from build123d import *

# Parameters (mm, degrees)
SKETCH_1_W          = 12
SKETCH_1_H          = 12
EXTRUDE_1_DEPTH     = 12
SKETCH_2_R          = 2
CUT_EXTRUDE_1_DEPTH = 21.784609691
SKETCH_3_R          = 2
CUT_EXTRUDE_2_DEPTH = 21.784609691
SKETCH_4_R          = 2
CUT_EXTRUDE_3_DEPTH = 21.784609691


with BuildPart() as part:
    # 草图1 → 凸台-拉伸1 (new body)
    with BuildSketch(Plane.XY):
        with Locations((6, -6)):
            Rectangle(SKETCH_1_W, SKETCH_1_H)
    extrude(amount=EXTRUDE_1_DEPTH)

    # 草图2 → 切除-拉伸1 (cut, through all)
    with BuildSketch(Plane(origin=(12, 0, 0), x_dir=(0, 0, -1), z_dir=(1, 0, 0))):
        with Locations(Location((-6, -6, 0), (0, 0, 90))):
            Circle(SKETCH_2_R)
    extrude(amount=-CUT_EXTRUDE_1_DEPTH, mode=Mode.SUBTRACT)

    # 草图3 → 切除-拉伸2 (cut, through all)
    with BuildSketch(Plane(origin=(0, 0, 0), x_dir=(1, 0, 0), z_dir=(0, 1, 0))):
        with Locations(Location((6, -6, 0), (0, 0, 270))):
            Circle(SKETCH_3_R)
    extrude(amount=-CUT_EXTRUDE_2_DEPTH, mode=Mode.SUBTRACT)

    # 草图4 → 切除-拉伸3 (cut, through all)
    with BuildSketch(Plane(origin=(0, 0, 0), x_dir=(-1, 0, 0), z_dir=(0, 0, -1))):
        with Locations((-6, -6)):
            Circle(SKETCH_4_R)
    extrude(amount=-CUT_EXTRUDE_3_DEPTH, mode=Mode.SUBTRACT)


solid = part.part
Geometry: final body of the model. Coordinates: model frame, mm. Round coordinates to 2 decimals unless told otherwise and drop trailing zeros. Loops run counter-clockwise (first coordinate to the right, second up) from the corner with the lowest first, then second, coordinate; pieces in that order, holes last. Notation, with made-up numbers: M 83.5,21 L 115.5,21 A25 ccw 115.5,41 Z; hole C -8,-29 d4. An arc over 180 degrees is marked long. Put each result on its own line as item: value. Start each with the question number.
(1) Draft query along X for faces 1 (the face through (3, -12, 6)), 2 (the face through (8, -6, 10)), 3 (the face through (12, -9, 6)). Return one class per face: +X half, -X half, draft (parallel to the pull), parting line (faces both ways), or undercut.
(2) Section query A-A (x = 3.75). Return loops of the section in (y, z), then the cut area to 3 significant figures.
(3) Section query B-B (z = 6.5). Return loops of the section in (x, y), then the cut area to 3 significant figures.
(4) Material intervals for line 1 along Y through (x, z) = (6, 1.9); line 2 along Z through (x, y) = (9.95, -6); line 3 along Y through (x, z) = (5.5, 4), sorted ascending. Write a range as [from, to].
(5) Section query D-D (y = -2.25). Return loops of the section in (x, z).
(6) Section query C-C (x = 6). Return loops of the section in (y, z), then the cut area to 3 significant figures.
Findings below:
1. face 1: draft
1. face 2: undercut
1. face 3: +X half
2. outline: M -12,0 L 0,0 L 0,12 L -12,12 Z; hole C -6,6 d4
2. area: 131 mm2
3. outline: M 0,-12 L 4.06,-12 L 4.06,-7.94 L 0,-7.94 Z; M 0,-4.06 L 4.06,-4.06 L 4.06,0 L 0,0 Z; M 7.94,-12 L 12,-12 L 12,-7.94 L 7.94,-7.94 Z; M 7.94,-4.06 L 12,-4.06 L 12,0 L 7.94,0 Z
3. area: 66.0 mm2
4. line 1: y = [-12, -8], [-4, 0]
4. line 2: z = [0, 4], [8, 12]
4. line 3: y = [-12, -7.94], [-4.06, 0]
5. outline: M 0,0 L 12,0 L 12,12 L 0,12 Z; hole C 6,6 d4
6. outline: M -12,0 L -8,0 L -8,4 L -12,4 Z; M -12,8 L -8,8 L -8,12 L -12,12 Z; M -4,0 L 0,0 L 0,4 L -4,4 Z; M -4,8 L 0,8 L 0,12 L -4,12 Z
6. area: 64.0 mm2
